from build123d import *


with BuildPart() as part:
    # Sketch → Revolution (revolve)
    with BuildSketch(Plane.YZ):
        Polygon((150, 0), (150, 25), (5, 25), (5, 70), (0, 70), (0, 0), align=None)
    revolution = revolve(axis=Axis((0, 0, 0), (0, 0, 1)))

    # Mirrored: Revolution across Sketch H_Axis
    add(revolution.mirror(Plane.XY))


solid = part.part
CAD build for the part. Positions are in the model's coordinates, mm. A direction names the side the tool comes from. Round coordinates to 2 decimals unless told otherwise and drop trailing zeros. Write each loop counter-clockwise with the first axis right and the second up, starting at its lowest first coordinate (ties: lowest second). Pieces come first, ordered by that corner, then holes. Notation, with made-up numbers: M -7,30.5 L 26,30.5 A24 cw 26,52.5 Z; hole C 62,-13.75 d11. An arc over 180 degrees is marked long. Put each result on its own line as item: value. Start each with the question number.
1) Saw through at C-C, the plane z = 51.5. Write the cut outline in (x, y).
2) Saw through at A-A, the plane x = 0. Write the cut outline in (y, z).
3) 3-axis set-ups, long thin cutter, end or side, ignore diameter. For faces 1 (the cylindrical face through (4.88, -1.08, 47.82)), 2 (the cylindrical face through (4.88, -1.08, -47.82)), 3 (the flat face through (0, 0, 70)): which of +Z, -Z, +X, -X, +Y, -Y reach the whole face in a straight line?
4) Pin check, flat tips, straight feed: pin 1 Ø1 at (x, y) = (-11.5, -46) entering from +Z; pin 2 Ø4 at (x, z) = (-80.5, -13) entering from +Y; pin 3 Ø3 at (y, z) = (-78, 1.5) entering from +X. Stop position of each tip, or through.
5) Drill centre lines: probe 1 along Z at (x, y) = (12, -63); probe 2 along Y at (x, z) = (53, -13); probe 3 along X at (y, z) = (-1, 12). Where is each one in solid material? Low to high. Write a range as [from, to].
6) Saw through at D-D, the plane z = 10.5. Write the cut outline in (x, y).
Resolved:
1. outline: C 0,0 d10
2. outline: M -150,-25 L -5,-25 L -5,-70 L 5,-70 L 5,-25 L 150,-25 L 150,25 L 5,25 L 5,70 L -5,70 L -5,25 L -150,25 Z
3. face 1: +Z
3. face 2: -Z
3. face 3: +Z, +X, -X, +Y, -Y
4. pin 1: z = 25
4. pin 2: y = 127.82
4. pin 3: x = 129.03
5. probe 1: [-25, 25]
5. probe 2: [-140.32, 140.32]
5. probe 3: [-150, 150]
6. outline: C 0,0 d300
